```python
from build123d import *

# Parameters (mm, degrees)
F1_DEPTH = 25.4
F2_DEPTH = 67.818
F3_DEPTH = 20.828
F4_DEPTH = 8.636


with BuildPart() as f1:
    # F0 (on Front) → F1 (new body)
    with BuildSketch(Plane.XZ):
        Polygon((54.8201352358, 0), (-5.1254355349, 0), (-5.1254355349, 34.9269658327), (-58.3828687668, 34.9269658327), (-58.3828687668, -37.4040566385), (54.8201352358, -37.4040566385), align=None)
    extrude(amount=F1_DEPTH)

    # F2 (add): a face of the model
    f2_faces = [f1.faces().sort_by_distance(p)[0] for p in [
        (-10.92964208, -25.4, -7.6636129895),
    ]]
    extrude(f2_faces, amount=F2_DEPTH)

    # F3 (cut): a face of the model
    f3_faces = [f1.faces().sort_by_distance(p)[0] for p in [
        (-10.92964208, -93.218, -7.6636129895),
    ]]
    extrude(f3_faces, amount=-F3_DEPTH, mode=Mode.SUBTRACT)

    # F4 (cut): a face of the model
    f4_faces = [f1.faces().sort_by_distance(p)[0] for p in [
        (54.8201352358, -36.195, -18.7020283192),
    ]]
    extrude(f4_faces, amount=-F4_DEPTH, mode=Mode.SUBTRACT)


solid = f1.part
```
Build history of the part. All positions in model axes, mm. A direction names the side the tool comes from. Round coordinates to 2 decimals unless told otherwise and drop trailing zeros. Write each loop counter-clockwise with the first axis right and the second up, starting at its lowest first coordinate (ties: lowest second). Pieces come first, ordered by that corner, then holes.
1) Drill centre lines: probe 1 along X at (y, z) = (-43.5, 9.5); probe 2 along Z at (x, y) = (1.5, -67). Where is each one in solid material? Low to high.
2) Pin check, flat tips, straight feed: pin 1 (15.5 mm diameter, centred on x = 9, y = -19.5, fed in from +Z); pin 2 (2 mm diameter, centred on y = -33, z = 13.5, fed in from +X). Stop position of each tip, or through.
3) Band-saw the part on C-C, the plane x = 34. List the corners of the cut face in (y, z).
4) Band-saw the part on A-A, the plane z = 18.5. List the corners of the cut face in (x, y), and give its area (3 significant figures).
5) 3-axis set-ups, long thin cutter, end or side, ignore diameter. For faces 1 (the flat face through (-18, 0, -9)), 2 (the flat face through (21, -36, 0)): which of +Z, -Z, +X, -X, +Y, -Y reach the whole face in a straight line?
6) Band-saw the part on B-B, the plane y = -27. List the corners of the cut face in (x, z).
Ans:
1. probe 1: x = -58.38 to -5.13
1. probe 2: z = -37.4 to 0
2. pin 1: stops at z = 0
2. pin 2: stops at x = -5.13
3. outline: (-72.39, -37.4) - (0, -37.4) - (0, 0) - (-72.39, 0) - close
4. outline: (-58.38, -72.39) - (-5.13, -72.39) - (-5.13, 0) - (-58.38, 0) - close
4. area: 3,860 mm2
5. face 1: +Z, -Z, +X, -X, +Y
5. face 2: +Z, +X, +Y, -Y
6. outline: (-58.38, -37.4) - (46.18, -37.4) - (46.18, 0) - (-5.13, 0) - (-5.13, 34.93) - (-58.38, 34.93) - close
